Input: part model. Units: mm. Frame: model coordinates. Round coordinates to 2 decimals unless told otherwise and drop trailing zeros. Order: outer loops, then holes, each group sorted by start corner. A loop starts at its lowest first (then second) coordinate and runs counter-clockwise, first axis right, second up. Notation, with made-up numbers: (37, 60.25) - (68, 60.25) arc R38 ccw to (68, 98.25) - close; hole circle Ø8 at (19.25, 78.5). An arc over 180 degrees is marked (long way). One line per item, written item: value. Start each with the question number.
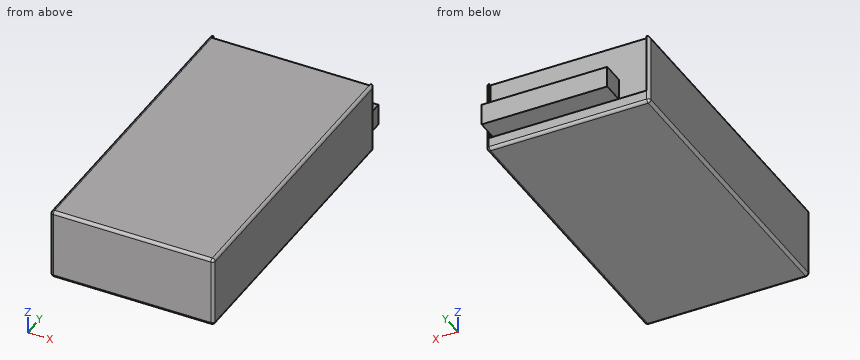
from build123d import *

# Parameters (mm, degrees)
F0_W     = 115
F0_H     = 215
F1_DEPTH = 25
F2_W     = 111
F2_H     = 41.5
F3_DEPTH = 2
F4_W     = 88.5
F4_H     = 15
F5_DEPTH = 16
F6_R     = 1.99999


# Not quite as in the source:
# - a fillet or chamfer is up to 0.001 mm smaller than in the source, because OpenCascade refuses the exact size


with BuildPart() as f1:
    # F0 (on Top) → F1 (new body, symmetric)
    with BuildSketch(Plane.XY):
        Rectangle(F0_W, F0_H)
    extrude(amount=F1_DEPTH, both=True)

    # F2 (on face) → F3 (cut)
    with BuildSketch(Plane(origin=(0, 107.5, 0), x_dir=(-1, 0, 0), z_dir=(0, 1, 0))):
        with Locations((0, 4.25)):
            Rectangle(F2_W, F2_H)
    extrude(amount=-F3_DEPTH, mode=Mode.SUBTRACT)

    # F4 (on face) → F5 (join)
    with BuildSketch(Plane(origin=(0, 105.5, 0), x_dir=(-1, 0, 0), z_dir=(0, 1, 0))):
        with Locations((-9.25, -8)):
            Rectangle(F4_W, F4_H)
    extrude(amount=F5_DEPTH)

    # F6 (radius 2 in the source; OpenCascade refuses exactly that, so slightly less here)
    f6_edges = [f1.edges().sort_by_distance(p)[0] for p in [
        (-57.5, 107.5, 0),
        (-57.5, 0, -25),
        (-57.5, -107.5, 0),
        (-57.5, 0, 25),
        (57.5, 0, -25),
        (57.5, 107.5, 0),
        (57.5, 0, 25),
        (57.5, -107.5, 0),
        (0, 107.5, -25),
        (0, -107.5, -25),
        (0, -107.5, 25),
    ]]
    fillet(f6_edges, radius=F6_R)


solid = f1.part
1. Section C-C (x = -49). Return the cut outline in (y, z), then the cut area to 3 significant figures.
2. Pin query (flat end, axial travel): pin 1 (2 mm diameter, centred on y = 107, z = 9, fed in from -X); pin 2 (1 mm diameter, centred on x = 34, z = -20, fed in from +Y); pin 3 (17.5 mm diameter, centred on x = 23.5, y = 114.5, fed in from -Z). Return the tip coordinate at first contact, or that it passes through.
3. Section B-B (x = -18.5). Return the cut outline in (y, z), then the cut area to 3 significant figures.
4. Line query: line 1 (Y direction, x = -38.5, z = -16); line 2 (Y direction, x = 6, z = -18). Output: solid intervals per line, ascending. Write a range as from..to.
Solved:
1. outline: (-107.5, -23) arc R2 ccw to (-105.5, -25) - (105.5, -25) arc R2 ccw to (107.5, -23) - (107.5, -16.5) - (105.5, -16.5) - (105.5, 25) - (-105.5, 25) arc R2 ccw to (-107.5, 23) - close
1. area: 10,700 mm²
2. pin 1: stops at x = -57.44
2. pin 2: stops at y = 107.5
2. pin 3: stops at z = -24.98
3. outline: (-107.5, -23) arc R2 ccw to (-105.5, -25) - (105.5, -25) arc R2 ccw to (107.5, -23) - (107.5, -16.5) - (105.5, -16.5) - (105.5, -15.5) - (121.5, -15.5) - (121.5, -0.5) - (105.5, -0.5) - (105.5, 25) - (-105.5, 25) arc R2 ccw to (-107.5, 23) - close
3. area: 10,900 mm²
4. line 1: y = -107.5..105.5
4. line 2: y = -107.5..107.5
